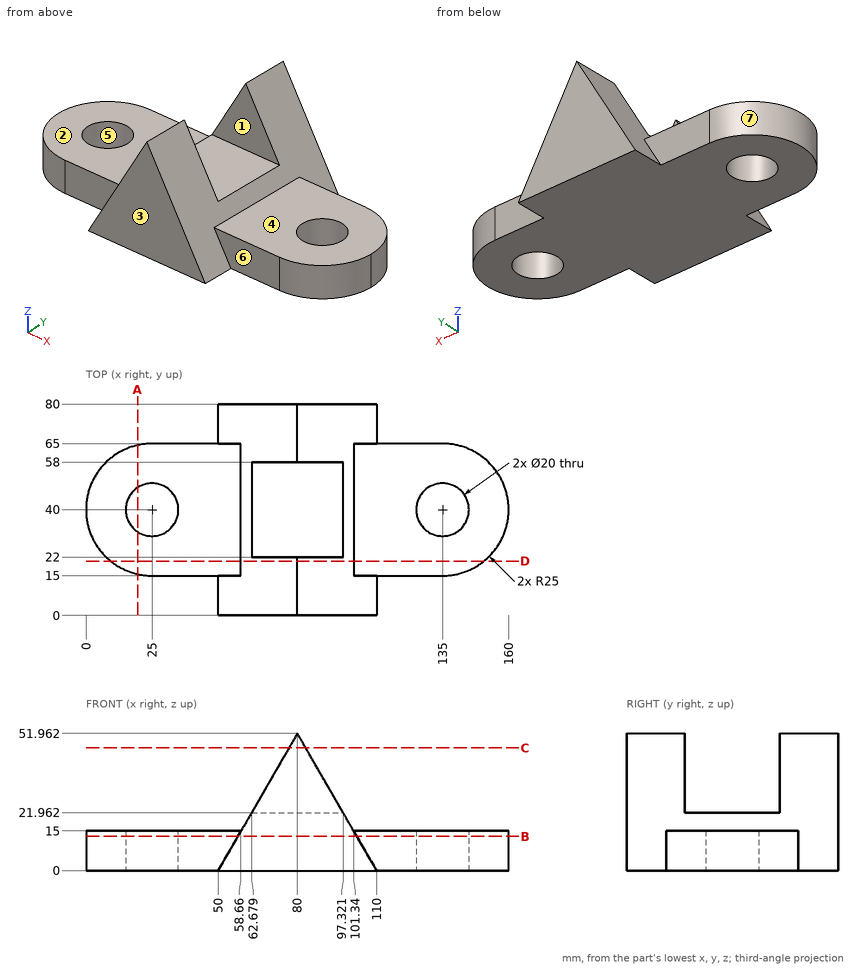
The figure shows three views and two pictorial views of one solid part (mm, origin at its lowest corner). Answer the questions. A direction names the side the tool comes from. Give positions to 0.01 mm unless a question says otherwise; leave off trailing zeros. Write each loop counter-clockwise with the first axis right and the second up, starting at its lowest first coordinate (ties: lowest second). Pieces come first, ordered by that corner, then holes. Notation, with made-up numbers: (28, -0.75) - (46, -0.75) arc R16 cw to (46, 9.25) - close; hole circle Ø8 at (52, 37). An arc over 180 degrees is marked (long way). Use CSV: the item, a comma, the result in double quotes. Start each with the question number.
Item 1: The part is cut by section A-A, the plane x = 19.5. Give the vertices of the cut face in (y, z).
Item 2: The part is cut by section B-B, the plane z = 13. Give the vertices of the cut face in (x, y) (1 decimal).
Item 3: The mould has two halves that part along X. Classify the marked faces 5, 6 and 7: pulls with the +X half, pulls with the -X half, needs draft (parallel to the pull), parting line crosses it, or undercut.
Item 4: Consider line 1 (Y direction, x = 135, z = 6); line 2 (Y direction, x = 32.5, z = 11.5) (1 decimal); line 3 (Z direction, x = 138.5, y = 58.5). Determine where each line is inside the solid, lowest interval first.
Item 5: The part is cut by section D-D, the plane y = 20.5. Give the vertices of the cut face in (x, z) (1 decimal).
Item 6: The part is cut by section C-C, the plane z = 46.5. Give the vertices of the cut face in (x, y).
Item 7: For the marked faces 1, 2, 3 and 4, determine the directions among +Z, -Z, +X, -X, +Y, -Y from which every point of the face is accessible in a straight line to the end or side of a thin tool.
Item 8: Flat-ended cylindrical pins translate along their axes: P1, Ø7.5, axis at x = 46, z = 5.5, coming from the -Y side; P2, Ø12, axis at x = 135, y = 40, coming from the -Z side; P3, Ø23, axis at x = 25, y = 40, coming from the -Z side; P4, Ø4.5, axis at x = 37, z = 6, coming from the +Y side. Find the tip coordinate at first contact, or state that the pin passes through.
Taken from the geometry:
1,outline,"(15.61, 0) - (31.65, 0) - (31.65, 15) - (15.61, 15) - close; (48.35, 0) - (64.39, 0) - (64.39, 15) - (48.35, 15) - close"
2,outline,"(25, 15) - (57.5, 15) - (57.5, 0) - (102.5, 0) - (102.5, 15) - (135, 15) arc R25 ccw to (135, 65) - (102.5, 65) - (102.5, 80) - (57.5, 80) - (57.5, 65) - (25, 65) arc R25 ccw to start; hole circle Ø20 at (25, 40); hole circle Ø20 at (135, 40)"
3,face 5,"undercut"
3,face 6,"needs draft"
3,face 7,"pulls with the -X half"
4,line 1,"15 to 30, 50 to 65"
4,line 2,"15 to 33.4, 46.6 to 65"
4,line 3,"0 to 15"
5,outline,"(9.4, 0) - (150.6, 0) - (150.6, 15) - (101.3, 15) - (80, 52) - (58.7, 15) - (9.4, 15) - close"
6,outline,"(76.85, 0) - (83.15, 0) - (83.15, 22) - (76.85, 22) - close; (76.85, 58) - (83.15, 58) - (83.15, 80) - (76.85, 80) - close"
7,face 1,"+Z, +X, -X"
7,face 2,"+Z, -X, +Y, -Y"
7,face 3,"+Z, -Z, +X, -X, -Y"
7,face 4,"+Z, +X, +Y, -Y"
8,P1,"y = 15"
8,P2,"through"
8,P3,"z = 0"
8,P4,"y = 65"
